```python
from build123d import *

# Parameters (mm, degrees)
SKETCH1_W                               = 18
SKETCH1_H                               = 100
BASE_DEPTH                              = 500
SKETCH2_W                               = 111
SKETCH2_H                               = 50
LAP_JOINT_CUTOUT_DEPTH                  = 511.219560582
LAP_JOINT_BOLT_HOLE_PATTERN_D           = 5.5
LAP_JOINT_BOLT_HOLE_PATTERN_CBORE_D     = 10
LAP_JOINT_BOLT_HOLE_PATTERN_CBORE_DEPTH = 5
CHAMFER_FRONT_SIZE                      = 176.5
CHAMFER_FRONT_SIZE2                     = 82.303301664
CHAMFER_REAR_SIZE                       = 176.5
CHAMFER_REAR_SIZE2                      = 82.303301664
BREAK_CHAMFER_OUTER_CORNERS_R           = 20
CROSS_TIE_BOLT_HOLE_PATTERN_D           = 5.5
CROSS_TIE_BOLT_HOLE_PATTERN_CBORE_D     = 10
CROSS_TIE_BOLT_HOLE_PATTERN_CBORE_DEPTH = 5
FILLET1_R                               = 10


with BuildPart() as part:
    # Sketch1 → base (new body)
    with BuildSketch(Plane.XY):
        with Locations((9, 50)):
            Rectangle(SKETCH1_W, SKETCH1_H)
    extrude(amount=BASE_DEPTH)

    # Sketch2 → lap joint cutout (cut, through all)
    with BuildSketch(Plane.ZY):
        with Locations((250, 75)):
            Rectangle(SKETCH2_W, SKETCH2_H)
    extrude(amount=-LAP_JOINT_CUTOUT_DEPTH, mode=Mode.SUBTRACT)

    # lap joint bolt hole pattern (through all)
    with Locations(Plane(origin=(18, 0, 0), x_dir=(0, 0, -1), z_dir=(1, 0, 0))):
        with Locations((-296.5, 40), (-203.5, 10), (-296.5, 10), (-203.5, 40)):
            CounterBoreHole(LAP_JOINT_BOLT_HOLE_PATTERN_D / 2, LAP_JOINT_BOLT_HOLE_PATTERN_CBORE_D / 2, LAP_JOINT_BOLT_HOLE_PATTERN_CBORE_DEPTH)

    # chamfer front
    chamfer_front_edges = [part.edges().sort_by_distance(p)[0] for p in [
        (9, 100, 0),
    ]]
    chamfer_front_side = [part.faces().sort_by_distance(p)[0] for p in [
        (9, 100, 97.25),
    ]]
    chamfer(chamfer_front_edges, length=CHAMFER_FRONT_SIZE, length2=CHAMFER_FRONT_SIZE2, reference=chamfer_front_side[0])

    # chamfer rear
    chamfer_rear_edges = [part.edges().sort_by_distance(p)[0] for p in [
        (9, 100, 500),
    ]]
    chamfer_rear_side = [part.faces().sort_by_distance(p)[0] for p in [
        (9, 100, 402.75),
    ]]
    chamfer(chamfer_rear_edges, length=CHAMFER_REAR_SIZE, length2=CHAMFER_REAR_SIZE2, reference=chamfer_rear_side[0])

    # break chamfer outer corners
    break_chamfer_outer_corners_edges = [part.edges().sort_by_distance(p)[0] for p in [
        (9, 17.696698336, 0),
        (9, 17.696698336, 500),
    ]]
    fillet(break_chamfer_outer_corners_edges, radius=BREAK_CHAMFER_OUTER_CORNERS_R)

    # cross tie bolt hole pattern (through all)
    with Locations(Plane(origin=(18, 0, 0), x_dir=(0, 0, -1), z_dir=(1, 0, 0))):
        with Locations((-314.5, 40), (-314.5, 10)):
            cross_tie_bolt_hole_pattern = CounterBoreHole(CROSS_TIE_BOLT_HOLE_PATTERN_D / 2, CROSS_TIE_BOLT_HOLE_PATTERN_CBORE_D / 2, CROSS_TIE_BOLT_HOLE_PATTERN_CBORE_DEPTH)

    # mirror cross tie bolt hole pattern: cross tie bolt hole pattern across plane
    add(cross_tie_bolt_hole_pattern.mirror(Plane(origin=(0, 0, 250), x_dir=(1, 0, 0), z_dir=(0, 0, -1))), mode=Mode.SUBTRACT)

    # Fillet1
    fillet1_edges = [part.edges().sort_by_distance(p)[0] for p in [
        (9, 100, 176.5),
        (9, 100, 323.5),
    ]]
    fillet(fillet1_edges, radius=FILLET1_R)


solid = part.part
```
Model file for the job. Use its own axes, mm. A direction names the side the tool comes from. Coordinates: 2 decimals unless noted, no trailing zeros. Write each loop counter-clockwise with the first axis right and the second up, starting at its lowest first coordinate (ties: lowest second). Pieces come first, ordered by that corner, then holes. Notation, with made-up numbers: (25, 56) - (42, 56) arc R8 cw to (42, 65) - close; hole circle Ø6 at (-18, 24.25). An arc over 180 degrees is marked (long way). One line per question, with ' | ' between items. Start each with the question number.
Q1. Pull direction Z, two halves, no side cores. Call faces 1 (the face through (9.13, 15.57, 496.95)), 2 (the face through (9, 100, 186)), 3 (the face through (13, 38, 201)): pulls with the +Z half, pulls with the -Z half, needs draft (parallel to the pull), parting line crosses it, or undercut.
Q2. Drill centre lines: line 1 (Y direction, x = 16.8, z = 203.5); line 2 (Y direction, x = 10.25, z = 296.5); line 3 (Y direction, x = 13.5, z = 262). Where is each one in solid material? Low to high. Write a range as [from, to].
Q3. Cut at B-B, the plane y = 57. List the corners of the cut face in (x, z).
Q4. Cut at C-C, the plane z = 443.5. List the corners of the cut face in (x, y), then the cut area to 3 significant figures.
Q5. Cut at A-A, the plane x = 3.5. Give the number of separate pieces and of enclosed holes in the cut face, then the cut area to 3 significant figures.
Q6. Pin check, flat tips, straight feed: pin 1 (1 mm diameter, centred on x = 13.5, z = 78.5, fed in from +Y) (3 decimals); pin 2 (8 mm diameter, centred on x = 12, y = 20, fed in from -Z); pin 3 (4 mm diameter, centred on x = 5, y = 84.5, fed in from +Z). Stop position of each tip, or through.
Q7. 3-axis set-ups, long thin cutter, end or side, ignore diameter. For faces 4 (the face through (13, 8, 201)), 5 (the face through (9, 100, 313)), 6 (the face through (9, 75, 194.5)): which of +Z, -Z, +X, -X, +Y, -Y reach the whole face in a straight line?
Q8. Cut at D-D, the plane y = 87. List the corners of the cut face in (x, z), then the cut area to 3 significant figures.
Answer below:
1) face 1: pulls with the +Z half | face 2: needs draft | face 3: undercut
2) line 1: [0, 5], [15, 35], [45, 50] | line 2: [0, 7.25], [12.75, 37.25], [42.75, 50] | line 3: [0, 50]
3) outline: (0, 84.29) - (18, 84.29) - (18, 194.5) - (0, 194.5) - close; (0, 305.5) - (18, 305.5) - (18, 415.71) - (0, 415.71) - close
4) outline: (0, 0) - (18, 0) - (18, 44.04) - (0, 44.04) - close | area: 793 mm^2
5) separate pieces: 1 | enclosed holes: 8 | area: 29,700 mm^2
6) pin 1: y = 54.535 | pin 2: z = 3.33 | pin 3: z = 361.03
7) face 4: +X | face 5: +Z, -Z, +X, -X, +Y | face 6: +X, -X, +Y
8) outline: (0, 148.62) - (18, 148.62) - (18, 194.5) - (0, 194.5) - close; (0, 305.5) - (18, 305.5) - (18, 351.38) - (0, 351.38) - close | area: 1,650 mm^2
